from build123d import *

# Parameters (mm, degrees)
F0_W     = 150
F0_H     = 60
F1_DEPTH = 3
F2_W     = 3
F2_H     = 30
F3_DEPTH = 25
F4_W     = 17.5
F4_H     = 10
F4_W_2   = 85
F5_DEPTH = 10
F6_R     = 10
F7_R     = 4.99999


# Not quite as in the source:
# - a fillet or chamfer is up to 0.001 mm smaller than in the source, because OpenCascade refuses the exact size


with BuildPart() as f1:
    # F0 (on Top) → F1 (new body)
    with BuildSketch(Plane.XY):
        Rectangle(F0_W, F0_H)
    extrude(amount=F1_DEPTH)

    # F2 (on Top) → F3 (cut)
    with BuildSketch(Plane.XY):
        with Locations((-67, 0)):
            Rectangle(F2_W, F2_H)
        with Locations((-31.5, 0)):
            Rectangle(F2_W, F2_H)
        with Locations((-4, 0)):
            Rectangle(F2_W, F2_H)
        with Locations((4, 0)):
            Rectangle(F2_W, F2_H)
        with Locations((31.5, 0)):
            Rectangle(F2_W, F2_H)
        with Locations((67, 0)):
            Rectangle(F2_W, F2_H)
    extrude(amount=F3_DEPTH, mode=Mode.SUBTRACT)

    # F4 (on Top) → F5 (join)
    with BuildSketch(Plane.XY):
        with Locations((-66.25, 25)):
            Rectangle(F4_W, F4_H)
        with Locations((66.25, 25)):
            Rectangle(F4_W, F4_H)
        with Locations((-66.25, -25)):
            Rectangle(F4_W, F4_H)
        with Locations((66.25, -25)):
            Rectangle(F4_W, F4_H)
        with Locations((0, 25)):
            Rectangle(F4_W_2, F4_H)
        with Locations((0, -25)):
            Rectangle(F4_W_2, F4_H)
    extrude(amount=-F5_DEPTH)

    # F6
    f6_edges = [f1.edges().sort_by_distance(p)[0] for p in [
        (-75, 30, -3.5),
        (-75, -30, -3.5),
        (75, -30, -3.5),
        (75, 30, -3.5),
    ]]
    fillet(f6_edges, radius=F6_R)

    # F7 (radius 5 in the source; OpenCascade refuses exactly that, so slightly less here)
    f7_edges = [f1.edges().sort_by_distance(p)[0] for p in [
        (57.5, 20, -5),
        (42.5, 20, -5),
        (57.5, -20, -5),
        (42.5, -20, -5),
        (42.5, -30, -5),
        (57.5, -30, -5),
        (57.5, 30, -5),
        (42.5, 30, -5),
        (-42.5, 20, -5),
        (-42.5, -30, -5),
        (-42.5, -20, -5),
        (-57.5, -20, -5),
        (-57.5, -30, -5),
        (-57.5, 20, -5),
        (-42.5, 30, -5),
        (-57.5, 30, -5),
    ]]
    fillet(f7_edges, radius=F7_R)


solid = f1.part
Could you check a few things on this model? Use its own coordinates, in mm. A direction names the side the tool comes from. Round coordinates to 2 decimals unless told otherwise and drop trailing zeros. Order: outer loops, then holes, each group sorted by start corner. A loop starts at its lowest first (then second) coordinate and runs counter-clockwise, first axis right, second up.
(1) Imagine slicing it at A-A (y = 3.5). Write out the boundary of the cut face in (x, z), plus the area to 3 significant figures.
Response values:
outline: (-75, 0) - (-68.5, 0) - (-68.5, 3) - (-75, 3) - close; (-65.5, 0) - (-33, 0) - (-33, 3) - (-65.5, 3) - close; (-30, 0) - (-5.5, 0) - (-5.5, 3) - (-30, 3) - close; (-2.5, 0) - (2.5, 0) - (2.5, 3) - (-2.5, 3) - close; (5.5, 0) - (30, 0) - (30, 3) - (5.5, 3) - close; (33, 0) - (65.5, 0) - (65.5, 3) - (33, 3) - close; (68.5, 0) - (75, 0) - (75, 3) - (68.5, 3) - close
area: 396 mm2
(2) Imagine slicing it at B-B (z = 1.5). Count the separate pieces of the cut face and the enclosed holes in it, plus the area to 3 significant figures.
Response values:
separate pieces: 1
enclosed holes: 6
area: 8,370 mm2
(3) If we mould it in two halves opening along X, with no side actions, what happens to faces 5 (the cylindrical face through (72.15, -26.99, -3.41)), 6 (the flat face through (-1, -20, -5)), 7 (the cylindrical face through (41.07, -21.5, -5.07))? For each: released by +X, released by -X, zero draft, split by the parting line, or undercut.
Response values:
face 5: released by +X
face 6: zero draft
face 7: undercut
(4) Imagine slicing it at C-C (x = 35.5). Write out the boundary of the cut face in (y, z), plus the area to 3 significant figures.
Response values:
outline: (-30, -10) - (-20, -10) - (-20, 0) - (20, 0) - (20, -10) - (30, -10) - (30, 3) - (-30, 3) - close
area: 380 mm2
(5) Which directions (+Z, -Z, +X, -X, +Y, -Y) give clear straight access to the entire face, cutting with the end or side of a thin tool? Please do faces 1 (the flat face through (-69, -20, -5)), 2 (the flat face through (-32, -15, 1)), 3 (the cylindrical face through (41, -28.57, -5.07)), 4 (the cylindrical face through (-59, 21.43, -5.07)).
Response values:
face 1: -Z, +X, -X
face 2: +Z, -Z
face 3: -Z, -Y
face 4: -Z
(6) I'm going to push flat-ended pins straight in: pin 1 (3 mm diameter, centred on x = -68.5, z = -3.5, fed in from -Y); pin 2 (2.5 mm diameter, centred on x = -67.5, z = 1, fed in from +Y); pin 3 (5 mm diameter, centred on x = 44, y = 5, fed in from -Z). Where does each tip first touch, or does it pass through?
Response values:
pin 1: stops at y = -29.8
pin 2: stops at y = 29.92
pin 3: stops at z = 0
(7) Please list where these lines run through material, in increasing order: line 1 along Y through (x, z) = (-37, -3); line 2 along X through (y, z) = (22, -5.75); line 3 along X through (y, z) = (-21, -4).
Response values:
line 1: y = -30 to -20, 20 to 30
line 2: x = -74.8 to -58.5, -41.5 to 41.5, 58.5 to 74.8
line 3: x = -74.95 to -59.5, -40.5 to 40.5, 59.5 to 74.95
